Check sheet for the drawn part. Datum: minimum x, y, z corner. Units: mm. A direction names the side the tool comes from. Coordinates: 2 decimals unless noted, no trailing zeros. Loops run counter-clockwise (first coordinate to the right, second up) from the corner with the lowest first, then second, coordinate; pieces in that order, holes last. Notation, with made-up numbers: (33, 8.25) -> (87, 8.25) arc R16 ccw to (87, 39.25) -> close; hole circle Ø4 at (78.5, 45). An arc over 180 degrees is marked (long way). Use CSV: the item, a comma, the result in double quotes. Start each with the question number.
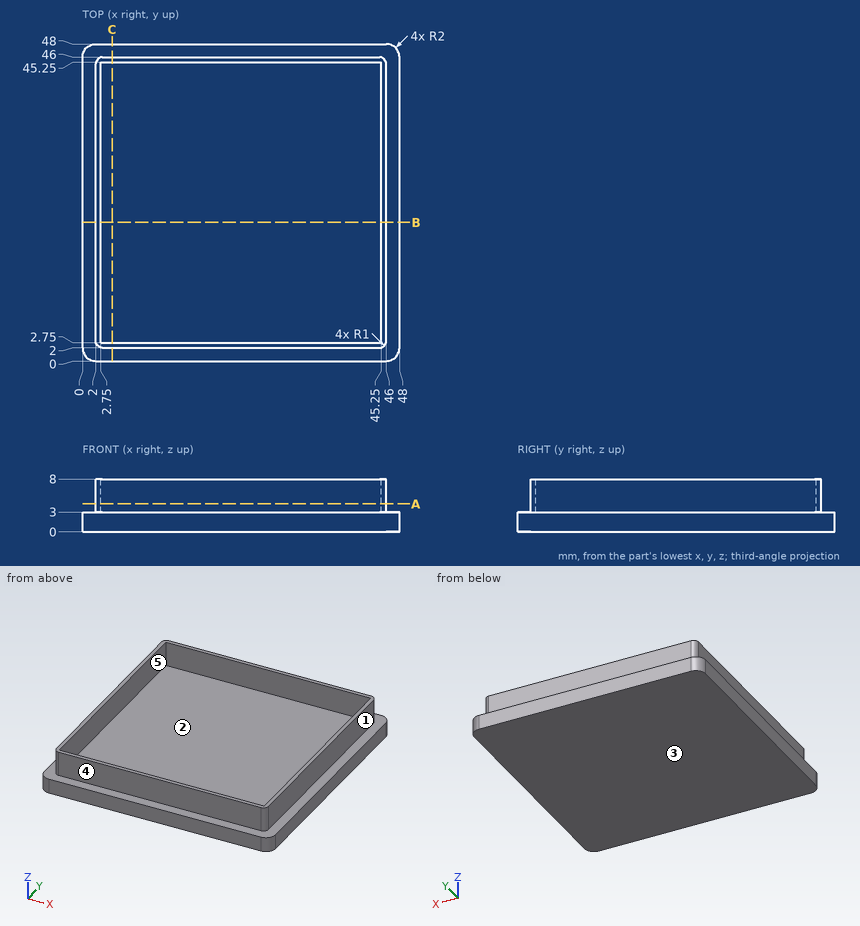
1. Depth check by flat-ended pin: pin 1 (24 mm diameter, centred on x = 29, y = 22, fed in from +Z); pin 2 (4 mm diameter, centred on y = 19.5, z = 5.5, fed in from -X); pin 3 (1.5 mm diameter, centred on y = 29.5, z = 6.5, fed in from +X). Enter the tip coordinate at first touch or a pass-through.
2. Set-up check for the marked faces 4 and 5: record each of +Z, -Z, +X, -X, +Y, -Y from which the full face is reachable in a straight line by a thin tool's end or side.
3. Release check for a two-part mould opening along Z. For the marked faces 1, 2 and 3 record: released by +Z, released by -Z, zero draft, split by the parting line, or undercut.
4. Scan lines: line 1 (Y direction, x = 41.5, z = 5.75); line 2 (Z direction, x = 20.5, y = 30). Record each from-to range of solid material in increasing order.
5. Cross-section at A-A, the plane z = 4.25. Record the boundary of the cut face in (x, y), plus the area to 3 significant figures.
6. Cross-section at B-B, the plane y = 21. Record the boundary of the cut face in (x, z).
Solution:
1,pin 1,"stops at z = 3"
1,pin 2,"stops at x = 2"
1,pin 3,"stops at x = 46"
2,face 4,"+Z, +X, -X, -Y"
2,face 5,"+Z"
3,face 1,"zero draft"
3,face 2,"released by +Z"
3,face 3,"released by -Z"
4,line 1,"y = 2 to 2.75, 45.25 to 46"
4,line 2,"z = 0 to 3"
5,outline,"(2, 3) arc R1 ccw to (3, 2) -> (45, 2) arc R1 ccw to (46, 3) -> (46, 45) arc R1 ccw to (45, 46) -> (3, 46) arc R1 ccw to (2, 45) -> close; hole (2.75, 2.75) -> (45.25, 2.75) -> (45.25, 45.25) -> (2.75, 45.25) -> close"
5,area,"129 mm2"
6,outline,"(0, 0) -> (48, 0) -> (48, 3) -> (46, 3) -> (46, 8) -> (45.25, 8) -> (45.25, 3) -> (2.75, 3) -> (2.75, 8) -> (2, 8) -> (2, 3) -> (0, 3) -> close"
